from build123d import *

# Parameters (mm, degrees)
PAD001_DEPTH = 26
FILLET_R     = 5
THICKNESS_T  = -2
SKETCH010_R  = 2.5
PAD004_DEPTH = 11


with BuildPart() as part:
    # Sketch002 → Pad001 (new body)
    with BuildSketch(Plane.XY):
        with BuildLine():
            Line((10, 0), (140, 0))
            ThreePointArc((140, 0), (147.071068, 2.928932), (150, 10))
            Line((150, 10), (150, 40))
            ThreePointArc((150, 40), (147.071068, 47.071068), (140, 50))
            Line((140, 50), (10, 50))
            ThreePointArc((10, 50), (2.928932, 47.071068), (0, 40))
            Line((0, 40), (0, 10))
            ThreePointArc((0, 10), (2.928932, 2.928932), (10, 0))
        make_face()
    extrude(amount=PAD001_DEPTH)

    # Fillet
    fillet_edges = [part.edges().sort_by_distance(p)[0] for p in [
        (75, 0, 0),
    ]]
    fillet(fillet_edges, radius=FILLET_R)

    # Thickness
    thickness_openings = [part.faces().sort_by_distance(p)[0] for p in [
        (75, 25, 26),
    ]]
    offset(amount=THICKNESS_T, openings=thickness_openings)

    # Sketch010 (on Face28 of Thickness) → Pad004 (join)
    with BuildSketch(Plane.XY.offset(2)):
        with Locations((52, 37.5)):
            Circle(SKETCH010_R)
        with Locations((92.5, 36.8)):
            Circle(SKETCH010_R)
        with Locations((121, 11.2)):
            Circle(SKETCH010_R)
        with Locations((31, 11.2)):
            Circle(SKETCH010_R)
    extrude(amount=PAD004_DEPTH)


solid = part.part
Read the model definition and answer for the solid it produces. Units are mm, in the model's axes. A direction names the side the tool comes from. Give positions to 0.01 mm unless a question says otherwise; leave off trailing zeros. Loops run counter-clockwise (first coordinate to the right, second up) from the corner with the lowest first, then second, coordinate; pieces in that order, holes last. Notation, with made-up numbers: M -2.75,79.25 L 34.25,79.25 A24 ccw 34.25,115.25 Z; hole C -26,-5 d8. An arc over 180 degrees is marked long. Write each question's results on one line, items separated by ' | '.
1. Section D-D on y = 29.5 is taken. Give the vertices of the cut face in (x, z), plus the area to 3 significant figures.
Values:
outline: M 0,5 A5 ccw 5,0 L 145,0 A5 ccw 150,5 L 150,26 L 148,26 L 148,5 A3 cw 145,2 L 5,2 A3 cw 2,5 L 2,26 L 0,26 Z | area: 389 mm^2
2. Straight lines are drawn through the part: line 1 (Y direction, x = 46, z = 17); line 2 (X direction, y = 35, z = 14.25); line 3 (X direction, y = 39.5, z = 10). For each, find the intervals that lie inside material, in ascending order. Write a range as [from, to].
Values:
line 1: y = [0, 2], [48, 50] | line 2: x = [0, 2], [148, 150] | line 3: x = [0, 2], [50.5, 53.5], [148, 150]
3. The mould has two halves that part along Y. Classify faces 3 (the face through (3.01, 47.15, 15.35)), 4 (the face through (74, 0, 15)), 5 (the face through (149, 25, 2)), 6 (the face through (75.91, 2.86, 2.9)): pulls with the +Y half, pulls with the -Y half, needs draft (parallel to the pull), parting line crosses it, or undercut.
Values:
face 3: pulls with the +Y half | face 4: pulls with the -Y half | face 5: needs draft | face 6: undercut
4. Given pin 1 (12 mm diameter, centred on x = 73.5, y = 21.5, fed in from +Z); pin 2 (1.5 mm diameter, centred on x = 31, y = 12.5, fed in from +Z); pin 3 (3 mm diameter, centred on y = 5.5, z = 16.5, fed in from -X), each flat-ended and moving along its own axis, determine where each tip first touches the part or whether it passes through.
Values:
pin 1: stops at z = 2 | pin 2: stops at z = 13 | pin 3: stops at x = 0.46
5. Section C-C on z = 19.5 is taken. Give the vertices of the cut face in (x, y), plus the area to 3 significant figures.
Values:
outline: M 0,10 A10 ccw 10,0 L 140,0 A10 ccw 150,10 L 150,40 A10 ccw 140,50 L 10,50 A10 ccw 0,40 Z; hole M 2,10 A8 ccw 10,2 L 140,2 A8 ccw 148,10 L 148,40 A8 ccw 140,48 L 10,48 A8 ccw 2,40 Z | area: 753 mm^2
6. Section B-B on x = 41 is taken. Give the vertices of the cut face in (y, z), plus the area to 3 significant figures.
Values:
outline: M 0,5 A5 ccw 5,0 L 45,0 A5 ccw 50,5 L 50,26 L 48,26 L 48,5 A3 cw 45,2 L 5,2 A3 cw 2,5 L 2,26 L 0,26 Z | area: 189 mm^2
7. Section A-A on z = 8 is taken. Give the vertices of the cut face in (x, y).
Values:
outline: M 0,10 A10 ccw 10,0 L 140,0 A10 ccw 150,10 L 150,40 A10 ccw 140,50 L 10,50 A10 ccw 0,40 Z; C 31,11.2 d5; C 52,37.5 d5; C 92.5,36.8 d5; C 121,11.2 d5; hole M 2,10 A8 ccw 10,2 L 140,2 A8 ccw 148,10 L 148,40 A8 ccw 140,48 L 10,48 A8 ccw 2,40 Z
8. A tool of negligible diameter and unlimited length cuts with its end or side. For faces 1 (the face through (2, 25, 15)), 2 (the face through (150, 25, 15)), from which of +Z, -Z, +X, -X, +Y, -Y can it reach the whole face along a straight path? Write none if from no direction.
Values:
face 1: +Z | face 2: +Z, -Z, +X, +Y, -Y
